```python
from build123d import *

# Parameters (mm, degrees)
F1_DEPTH = 8.89
F2_DEPTH = 3.81


with BuildPart() as f1:
    # F0 (on Front) → F1 (new body)
    with BuildSketch(Plane.XZ):
        with BuildLine():
            Line((6.35, 0), (9.525, 0))
            ThreePointArc((9.525, 0), (8.248891971, 4.7625), (4.7625, 8.248891971))
            Line((4.7625, 8.248891971), (3.175, 5.499261314))
            ThreePointArc((3.175, 5.499261314), (5.499261314, 3.175), (6.35, 0))
        make_face()
        with BuildLine():
            Line((3.175, 5.499261314), (4.7625, 8.248891971))
            ThreePointArc((4.7625, 8.248891971), (0, 9.525), (-4.7625, 8.248891971))
            Line((-4.7625, 8.248891971), (-3.175, 5.499261314))
            ThreePointArc((-3.175, 5.499261314), (0, 6.35), (3.175, 5.499261314))
        make_face()
        with BuildLine():
            Line((4.7625, 0), (6.35, 0))
            ThreePointArc((6.35, 0), (5.499261314, 3.175), (3.175, 5.499261314))
            Line((3.175, 5.499261314), (2.38125, 4.1244459855))
            ThreePointArc((2.38125, 4.1244459855), (4.1244459855, 2.38125), (4.7625, 0))
        make_face()
        with BuildLine():
            Line((2.38125, 4.1244459855), (3.175, 5.499261314))
            ThreePointArc((3.175, 5.499261314), (0, 6.35), (-3.175, 5.499261314))
            Line((-3.175, 5.499261314), (-2.38125, 4.1244459855))
            ThreePointArc((-2.38125, 4.1244459855), (-1.8024489876, 4.4082404536), (-1.190625, 4.6112707966))
            Line((-1.190625, 4.6112707966), (-1.190625, 5.953125))
            Line((-1.190625, 5.953125), (1.190625, 5.953125))
            Line((1.190625, 5.953125), (1.190625, 4.6112707966))
            ThreePointArc((1.190625, 4.6112707966), (1.8024489876, 4.4082404536), (2.38125, 4.1244459855))
        make_face()
        with BuildLine():
            ThreePointArc((4.7625, -8.248891971), (8.248891971, -4.7625), (9.525, 0))
            Line((9.525, 0), (6.35, 0))
            ThreePointArc((6.35, 0), (5.499261314, -3.175), (3.175, -5.499261314))
            Line((3.175, -5.499261314), (4.7625, -8.248891971))
        make_face()
        with BuildLine():
            Line((-2.38125, 4.1244459855), (-3.175, 5.499261314))
            ThreePointArc((-3.175, 5.499261314), (-5.499261314, 3.175), (-6.35, 0))
            Line((-6.35, 0), (-4.7625, 0))
            ThreePointArc((-4.7625, 0), (-4.1244459855, 2.38125), (-2.38125, 4.1244459855))
        make_face()
        with BuildLine():
            ThreePointArc((-6.35, 0), (-5.499261314, -3.175), (-3.175, -5.499261314))
            Line((-3.175, -5.499261314), (-2.38125, -4.1244459855))
            ThreePointArc((-2.38125, -4.1244459855), (-4.1244459855, -2.38125), (-4.7625, 0))
            Line((-4.7625, 0), (-6.35, 0))
        make_face()
        with BuildLine():
            ThreePointArc((-9.525, 0), (-8.248891971, -4.7625), (-4.7625, -8.248891971))
            Line((-4.7625, -8.248891971), (-3.175, -5.499261314))
            ThreePointArc((-3.175, -5.499261314), (-5.499261314, -3.175), (-6.35, 0))
            Line((-6.35, 0), (-9.525, 0))
        make_face()
        with BuildLine():
            ThreePointArc((-4.7625, -8.248891971), (0, -9.525), (4.7625, -8.248891971))
            Line((4.7625, -8.248891971), (3.175, -5.499261314))
            ThreePointArc((3.175, -5.499261314), (0, -6.35), (-3.175, -5.499261314))
            Line((-3.175, -5.499261314), (-4.7625, -8.248891971))
        make_face()
        with BuildLine():
            ThreePointArc((-3.175, -5.499261314), (0, -6.35), (3.175, -5.499261314))
            Line((3.175, -5.499261314), (2.38125, -4.1244459855))
            ThreePointArc((2.38125, -4.1244459855), (0, -4.7625), (-2.38125, -4.1244459855))
            Line((-2.38125, -4.1244459855), (-3.175, -5.499261314))
        make_face()
        with BuildLine():
            ThreePointArc((3.175, -5.499261314), (5.499261314, -3.175), (6.35, 0))
            Line((6.35, 0), (4.7625, 0))
            ThreePointArc((4.7625, 0), (4.1244459855, -2.38125), (2.38125, -4.1244459855))
            Line((2.38125, -4.1244459855), (3.175, -5.499261314))
        make_face()
        with BuildLine():
            Line((-3.175, 5.499261314), (-4.7625, 8.248891971))
            ThreePointArc((-4.7625, 8.248891971), (-8.248891971, 4.7625), (-9.525, 0))
            Line((-9.525, 0), (-6.35, 0))
            ThreePointArc((-6.35, 0), (-5.499261314, 3.175), (-3.175, 5.499261314))
        make_face()
    extrude(amount=-F1_DEPTH)

    # F0 (on Front) → F2 (join)
    with BuildSketch(Plane.XZ):
        with BuildLine():
            Line((6.35, 0), (9.525, 0))
            ThreePointArc((9.525, 0), (8.248891971, 4.7625), (4.7625, 8.248891971))
            Line((4.7625, 8.248891971), (3.175, 5.499261314))
            ThreePointArc((3.175, 5.499261314), (5.499261314, 3.175), (6.35, 0))
        make_face()
        with BuildLine():
            ThreePointArc((-4.7625, -8.248891971), (0, -9.525), (4.7625, -8.248891971))
            Line((4.7625, -8.248891971), (3.175, -5.499261314))
            ThreePointArc((3.175, -5.499261314), (0, -6.35), (-3.175, -5.499261314))
            Line((-3.175, -5.499261314), (-4.7625, -8.248891971))
        make_face()
        with BuildLine():
            Line((-3.175, 5.499261314), (-4.7625, 8.248891971))
            ThreePointArc((-4.7625, 8.248891971), (-8.248891971, 4.7625), (-9.525, 0))
            Line((-9.525, 0), (-6.35, 0))
            ThreePointArc((-6.35, 0), (-5.499261314, 3.175), (-3.175, 5.499261314))
        make_face()
    extrude(amount=F2_DEPTH)


solid = f1.part
```
The listing builds one solid part. Answer for the finished solid, in the listing's coordinates (mm). A direction names the side the tool comes from. Give positions to 0.01 mm unless a question says otherwise; leave off trailing zeros. Order: outer loops, then holes, each group sorted by start corner. A loop starts at its lowest first (then second) coordinate and runs counter-clockwise, first axis right, second up. Notation, with made-up numbers: M -39,14.5 L 2,14.5 A29 ccw 2,53.5 Z; hole C -10.75,40.25 d11. An arc over 180 degrees is marked long. Put each result on its own line as item: value. Start each with the question number.
Item 1: For a pull along Z with two mould halves and no side action, classify faces 4 (the face through (0, 4, 5.953)), 5 (the face through (-2.3, 8.89, 4.4)), 6 (the face through (3.98, -1.88, 6.89)) as +Z half, -Z half, draft (parallel to the pull), parting line (faces both ways), or undercut.
Item 2: The part is cut by section A-A, the plane y = -1. State how many separate pieces and enclosed holes the cut face has, and give its area (3 significant figures).
Item 3: The part is cut by section D-D, the plane z = -1.75. Determine the outline of the cut face in (x, y).
Item 4: Find the intervals of material crossed by line 1 along Z through (x, y) = (4, 1.5); line 2 along X through (y, z) = (-1, 1.75); line 3 along X through (y, z) = (2.5, -1.5), in increasing order.
Item 5: Flat-ended cylindrical pins translate along their axes: P1, Ø2.5, axis at x = 8.5, y = -2, coming from the -Z side; P2, Ø0.7, axis at y = 3, z = 5.5, coming from the +X side; P3, Ø4, axis at x = -4, y = 7.5, coming from the -Z side. Find the tip coordinate at first contact, or state that the pin passes through.
Item 6: The part is cut by section B-B, the plane x = -4. Determine the outline of the cut face in (y, z).
Item 7: Which of the six approach directions +Z, -Z, +X, -X, +Y, -Y give full straight-line access (tool end or side, diameter ignored) to faces 1 (the face through (-1.191, 4, 5)), 2 (the face through (3.98, -1.88, -6.89)), 3 (the face through (8, -2, 0))?
Answer key:
1. face 4: undercut
1. face 5: draft
1. face 6: +Z half
2. separate pieces: 3
2. enclosed holes: 0
2. area: 79.2 mm²
3. outline: M -9.36,0 L -4.43,0 L -4.43,8.89 L -9.36,8.89 Z; M 4.43,0 L 9.36,0 L 9.36,8.89 L 4.43,8.89 Z
4. line 1: z = -8.64 to -2.58, 2.58 to 8.64
4. line 2: x = -9.36 to -6.1, 6.1 to 9.36
4. line 3: x = -9.41 to -4.52, 4.52 to 9.41
5. P1: stops at z = 0
5. P2: stops at x = 8.01
5. P3: stops at z = -9.31
6. outline: M -3.81,-8.64 L 8.89,-8.64 L 8.89,-2.58 L 0,-2.58 L 0,-6.93 L -3.81,-6.93 Z; M -3.81,4.93 L 0,4.93 L 0,2.58 L 8.89,2.58 L 8.89,8.64 L 0,8.64 L 0,6.93 L -3.81,6.93 Z
7. face 1: +Y, -Y
7. face 2: +X, -Y
7. face 3: -Z, +X, -X, -Y
